Check sheet for the modelled part. Datum: model origin and axes. Units: mm. A direction names the side the tool comes from. Coordinates: 2 decimals unless noted, no trailing zeros. Loops run counter-clockwise (first coordinate to the right, second up) from the corner with the lowest first, then second, coordinate; pieces in that order, holes last.
from build123d import *

# Parameters (mm, degrees)
F1_DEPTH = 63.5
F0_W     = 27.6187203676
F0_H     = 19.05
F2_DEPTH = 25.4
F3_DEPTH = 7.9375


with BuildPart() as f1:
    # F0 (on Front) → F1 (new body, symmetric)
    with BuildSketch(Plane.XZ):
        Polygon((-41.275, 9.525), (-41.275, -9.525), (41.275, -9.525), (41.275, 9.525), (22.225, 9.525), align=None)
    extrude(amount=F1_DEPTH, both=True)

    # F0 (on Front) → F2 (join, symmetric)
    with BuildSketch(Plane.XZ):
        with BuildLine():
            Line((22.225, 9.525), (41.275, 9.525))
            Line((41.275, 9.525), (41.275, 27.0002))
            ThreePointArc((41.275, 27.0002), (45.9246798487, 38.2255201513), (57.15, 42.8752))
            Line((57.15, 42.8752), (58.1062796324, 42.8752))
            Line((58.1062796324, 42.8752), (58.1062796324, 61.9252))
            Line((58.1062796324, 61.9252), (57.15, 61.9252))
            ThreePointArc((57.15, 61.9252), (32.4542956671, 51.6959043329), (22.225, 27.0002))
            Line((22.225, 27.0002), (22.225, 9.525))
        make_face()
        with Locations((71.9156398162, 52.4002)):
            Rectangle(F0_W, F0_H)
    extrude(amount=F2_DEPTH, both=True)

    # F0 (on Front) → F3 (join, symmetric)
    with BuildSketch(Plane.XZ):
        with BuildLine():
            add(Edge.make_bspline(
                [(-41.275, 9.525), (-39.7970601916, 27.7465097606), (7.8009576537, 62.4250620604), (57.15, 61.9252)],
                knots=[0, 0, 0, 0, 111.5045361635, 111.5045361635, 111.5045361635, 111.5045361635], degree=3))
            Line((-41.275, 9.525), (22.225, 9.525))
            Line((22.225, 9.525), (22.225, 27.0002))
            ThreePointArc((22.225, 27.0002), (32.4542956671, 51.6959043329), (57.15, 61.9252))
        make_face()
    extrude(amount=F3_DEPTH, both=True)

    # F0 (on Front) → F4 (revolve)
    with BuildSketch(Plane.XZ):
        Polygon((85.725, 66.675), (85.725, 61.9252), (85.725, 42.8752), (85.725, 38.1), (108.9062796324, 38.1), (108.9062796324, 66.675), align=None)
    revolve(axis=Axis((85.725, 0, 52.4002), (0, 0, 1)))


solid = f1.part
(1) Section check B-B, the plane z = -3.5. Enter the section's corners in (x, y) (3 decimals).
(2) Scan lines: line 1 along Z through (x, y) = (-28, -29.5) (3 decimals); line 2 along X through (y, z) = (31.5, 8.5) (3 decimals); line 3 along Z through (x, y) = (65.5, -22.5). Record each from-to range of solid material in increasing order.
(3) Set-up check for faces 4 (the face through (62, 0, 61.925)), 5 (the face through (46, -25.4, 42)), 6 (the face through (-2, -7.938, 30)), 7 (the face through (-2, 7.938, 30)), 8 (the face through (45.8, -0.4, 38.1)): record each of +Z, -Z, +X, -X, +Y, -Y from which the full face is reachable in a straight line by a thin tool's end or side.
(4) Gauge pin test, flat ends, axial feed: P1, Ø3, axis at y = -15.5, z = 3, coming from the +X side (3 decimals); P2, Ø8.5, axis at x = 75, y = 6.5, coming from the -Z side; P3, Ø4, axis at x = 2.5, z = 44, coming from the +Y side. Record the tip position at first contact, or that the pin passes through.
(5) Draft check along X on faces 1 (the face through (85, 0, 66.675)), 2 (the face through (22.225, 17, 18)), 3 (the face through (62, 0, 42.875)). Enter one of: pulls with the +X half, pulls with the -X half, needs draft (parallel to the pull), parting line crosses it, or undercut.
(6) Section check A-A, the plane y = -49.5. Enter the section's corners in (x, z) (3 decimals), plus the area to 3 significant figures.
Determined:
1. outline: (-41.275, -63.5) - (41.275, -63.5) - (41.275, 63.5) - (-41.275, 63.5) - close
2. line 1: z = -9.525 to 9.525
2. line 2: x = -41.275 to 41.275
2. line 3: z = 42.88 to 61.93
3. face 4: +Z, -X
3. face 5: +Z, +X, -X, -Y
3. face 6: +Z, -X, -Y
3. face 7: +Z, -X, +Y
3. face 8: -Z, +Y, -Y
4. P1: stops at x = 41.275
4. P2: stops at z = 38.1
4. P3: stops at y = 7.94
5. face 1: needs draft
5. face 2: pulls with the -X half
5. face 3: undercut
6. outline: (-41.275, -9.525) - (41.275, -9.525) - (41.275, 9.525) - (-41.275, 9.525) - close
6. area: 1,570 mm2
